from build123d import *

# Parameters (mm, degrees)
SKETCH_8_R      = 2
SKETCH_8_R_2    = 1.5
EXTRUDE_1_DEPTH = 1.6


with BuildPart() as part:
    # 草图8 → 凸台-拉伸1 (new body)
    with BuildSketch(Plane.XZ):
        with BuildLine():
            Line((30.529437252, 84), (36.227922061, 89.69848481))
            ThreePointArc((36.227922061, 89.69848481), (36.935028843, 89.991378029), (37.642135624, 89.69848481))
            Line((37.642135624, 89.69848481), (53.19848481, 74.142135624))
            ThreePointArc((53.19848481, 74.142135624), (53.491378029, 73.435028843), (53.19848481, 72.727922061))
            Line((53.19848481, 72.727922061), (47.5, 67.029437252))
            ThreePointArc((47.5, 67.029437252), (42.297453968, 59.24327688), (40.470562748, 50.058874503))
            Line((40.470562748, 50.058874503), (40.470562748, 36))
            ThreePointArc((40.470562748, 36), (47.5, 19.029437252), (64.470562748, 12))
            Line((64.470562748, 12), (77.470562748, 12))
            ThreePointArc((77.470562748, 12), (78.17766953, 11.707106781), (78.470562748, 11))
            Line((78.470562748, 11), (78.470562748, -11))
            ThreePointArc((78.470562748, -11), (78.17766953, -11.707106781), (77.470562748, -12))
            Line((77.470562748, -12), (64.470562748, -12))
            ThreePointArc((64.470562748, -12), (47.5, -19.029437252), (40.470562748, -36))
            Line((40.470562748, -36), (40.470562748, -50.058874503))
            ThreePointArc((40.470562748, -50.058874503), (42.297453968, -59.24327688), (47.5, -67.029437252))
            Line((47.5, -67.029437252), (53.19848481, -72.727922061))
            ThreePointArc((53.19848481, -72.727922061), (53.491378029, -73.435028843), (53.19848481, -74.142135624))
            Line((53.19848481, -74.142135624), (37.642135624, -89.69848481))
            ThreePointArc((37.642135624, -89.69848481), (36.935028843, -89.991378029), (36.227922061, -89.69848481))
            Line((36.227922061, -89.69848481), (30.529437252, -84))
            ThreePointArc((30.529437252, -84), (22.74327688, -78.797453968), (13.558874503, -76.970562748))
            Line((13.558874503, -76.970562748), (-13.558874503, -76.970562748))
            ThreePointArc((-13.558874503, -76.970562748), (-22.74327688, -78.797453968), (-30.529437252, -84))
            Line((-30.529437252, -84), (-36.227922061, -89.69848481))
            ThreePointArc((-36.227922061, -89.69848481), (-36.935028843, -89.991378029), (-37.642135624, -89.69848481))
            Line((-37.642135624, -89.69848481), (-53.19848481, -74.142135624))
            ThreePointArc((-53.19848481, -74.142135624), (-53.491378029, -73.435028843), (-53.19848481, -72.727922061))
            Line((-53.19848481, -72.727922061), (-47.5, -67.029437252))
            ThreePointArc((-47.5, -67.029437252), (-42.297453968, -59.24327688), (-40.470562748, -50.058874503))
            Line((-40.470562748, -50.058874503), (-40.470562748, -36))
            ThreePointArc((-40.470562748, -36), (-47.5, -19.029437252), (-64.470562748, -12))
            Line((-64.470562748, -12), (-77.470562748, -12))
            ThreePointArc((-77.470562748, -12), (-78.17766953, -11.707106781), (-78.470562748, -11))
            Line((-78.470562748, -11), (-78.470562748, 11))
            ThreePointArc((-78.470562748, 11), (-78.17766953, 11.707106781), (-77.470562748, 12))
            Line((-77.470562748, 12), (-64.470562748, 12))
            ThreePointArc((-64.470562748, 12), (-47.5, 19.029437252), (-40.470562748, 36))
            Line((-40.470562748, 36), (-40.470562748, 50.058874503))
            ThreePointArc((-40.470562748, 50.058874503), (-42.297453968, 59.24327688), (-47.5, 67.029437252))
            Line((-47.5, 67.029437252), (-53.19848481, 72.727922061))
            ThreePointArc((-53.19848481, 72.727922061), (-53.491378029, 73.435028843), (-53.19848481, 74.142135624))
            Line((-53.19848481, 74.142135624), (-37.642135624, 89.69848481))
            ThreePointArc((-37.642135624, 89.69848481), (-36.935028843, 89.991378029), (-36.227922061, 89.69848481))
            Line((-36.227922061, 89.69848481), (-30.529437252, 84))
            ThreePointArc((-30.529437252, 84), (-22.74327688, 78.797453968), (-13.558874503, 76.970562748))
            Line((-13.558874503, 76.970562748), (13.558874503, 76.970562748))
            ThreePointArc((13.558874503, 76.970562748), (22.74327688, 78.797453968), (30.529437252, 84))
        make_face()
        with Locations(Location((-61.470562748, 8, 0), (0, 0, 90))):
            Circle(SKETCH_8_R, mode=Mode.SUBTRACT)
        with Locations(Location((-25.887975085, -10.446849588, 0), (0, 0, 90))):
            Circle(SKETCH_8_R_2, mode=Mode.SUBTRACT)
        with Locations(Location((-25.887975085, 64.387975085, 0), (0, 0, 90))):
            Circle(SKETCH_8_R_2, mode=Mode.SUBTRACT)
        with Locations(Location((-61.470562748, -8, 0), (0, 0, 90))):
            Circle(SKETCH_8_R, mode=Mode.SUBTRACT)
    extrude(amount=EXTRUDE_1_DEPTH)


solid = part.part
The listing builds one solid part. Answer for the finished solid, in the listing's coordinates (mm). A direction names the side the tool comes from. Coordinates: 2 decimals unless noted, no trailing zeros. Write each loop counter-clockwise with the first axis right and the second up, starting at its lowest first coordinate (ties: lowest second). Pieces come first, ordered by that corner, then holes. Notation, with made-up numbers: M 39.25,59 L 53.25,59 A24 ccw 53.25,97 Z; hole C -32,46.5 d10. An arc over 180 degrees is marked long. Put each result on its own line as item: value. Start each with the question number.
1. A cutting plane is placed at C-C on y = -1.05. Count the separate pieces of the cut face and the enclosed holes in it, then the cut area to 3 significant figures.
2. For a pull along X with two mould halves and no side action, classify faces 1 (the flat face through (33.42, -0.79, -86.89)), 2 (the flat face through (-50.31, -0.79, 69.84)), 3 (the cylindrical face through (47.69, -0.79, -18.84)) as pulls with the +X half, pulls with the -X half, needs draft (parallel to the pull), parting line crosses it, or undercut.
3. A cutting plane is placed at B-B on x = -67.5. Write down the section's boundary in (y, z), then the cut area to 3 significant figures.
4. A cutting plane is placed at D-D on z = 27.5. Write down the section's boundary in (x, y), then the cut area to 3 significant figures.
5. Which of the six approach directions +Z, -Z, +X, -X, +Y, -Y give full straight-line access (tool end or side, diameter ignored) to faces 4 (the flat face through (-33.42, -0.79, 86.89)), 5 (the cylindrical face through (-47.31, -0.79, -19.22)), 6 (the cylindrical face through (22.87, -0.79, -78.85)), 7 (the cylindrical face through (42.247, -0.789, -59.121))?
6. Flat-ended cylindrical pins translate along their axes: P1, Ø0.8, axis at x = -6.5, y = -1, coming from the -Z side; P2, Ø0.5, axis at y = -0.5, z = -46, coming from the +X side; P3, Ø0.5, axis at x = -71, y = -0.5, coming from the +Z side. Find the tip coordinate at first contact, or state that the pin passes through.
7. A cutting plane is placed at A-A on z = 8. Write down the section's boundary in (x, y), then the cut area to 3 significant figures.
8. Consider line 1 (X direction, y = -0.9, z = 8); line 2 (Z direction, x = 47, y = -0.8); line 3 (Z direction, x = -47.5, y = -0.2). Determine where each line is inside the solid, lowest interval first. Write a range as from..to.
Resolved:
1. separate pieces: 1
1. enclosed holes: 4
1. area: 16,100 mm2
2. face 1: undercut
2. face 2: pulls with the -X half
2. face 3: pulls with the +X half
3. outline: M -1.6,-12 L 0,-12 L 0,12 L -1.6,12 Z
3. area: 38.4 mm2
4. outline: M -42.03,-1.6 L 42.03,-1.6 L 42.03,0 L -42.03,0 Z
4. area: 134 mm2
5. face 4: +Z, +Y, -Y
5. face 5: -X, +Y, -Y
5. face 6: -Z, +Y, -Y
5. face 7: +X, +Y, -Y
6. P1: stops at z = -76.97
6. P2: stops at x = 40.47
6. P3: stops at z = 12
7. outline: M -78.47,-1.6 L -63.47,-1.6 L -63.47,0 L -78.47,0 Z; M -59.47,-1.6 L 78.47,-1.6 L 78.47,0 L -59.47,0 Z
7. area: 245 mm2
8. line 1: x = -78.47..-63.47, -59.47..78.47
8. line 2: z = -80.34..-66.51, -19.54..19.54, 66.51..80.34
8. line 3: z = -79.84..-67.03, -19.03..19.03, 67.03..79.84
